Verification items for the finished model (mm, model axes). A direction names the side the tool comes from. Coordinates: 2 decimals unless noted, no trailing zeros. Order: outer loops, then holes, each group sorted by start corner. A loop starts at its lowest first (then second) coordinate and runs counter-clockwise, first axis right, second up.
Q1. Set-up check for faces 4 (the flat face through (0, 8, 49)), 5 (the flat face through (8, 0, 49)), 6 (the flat face through (8, -17, 49)), 7 (the flat face through (-5.05, -19, 49)): record each of +Z, -Z, +X, -X, +Y, -Y from which the full face is reachable in a straight line by a thin tool's end or side.
Q2. Cross-section at A-A, the plane x = 0. Record the boundary of the cut face in (y, z).
Q3. Thickness scan on line 1 (X direction, y = 0, z = 33); line 2 (X direction, y = 18.5, z = 95); line 3 (X direction, y = -8.5, z = 15). Record the ranges inside material, lowest first.
Q4. Depth check by flat-ended pin: P1, Ø8, axis at x = 0.5, z = 16.5, coming from the -Y side; P2, Ø5, axis at x = -15.5, y = 3, coming from the +Z side; P3, Ø5, axis at x = -0.5, z = 18, coming from the -Y side. Enter the tip coordinate at first touch or a pass-through.
Q5. Draft check along X on faces 1 (the flat face through (-19, 5.05, 49)), 2 (the flat face through (-20, 13, 49)), 3 (the flat face through (8.305, -11.134, 50.7)). Enter one of: pulls with the +X half, pulls with the -X half, needs draft (parallel to the pull), parting line crosses it, or undercut.
Autodesk Inventor part; units mm, degrees
ref_plane "YZ Plane" through (0, 0, 0) normal (1, 0, 0) x (0, 1, 0)
ref_plane "XZ Plane" through (0, 0, 0) normal (0, 1, 0) x (-1, 0, 0)
ref_plane "XY Plane" through (0, 0, 0) normal (0, 0, 1) x (1, 0, 0)
sketch "Sketch1" plane through (0, 0, 0) normal (0, 0, 1) x (1, 0, 0)
  arc A0 (0, 5) -> (-5, 0) centre (0, 0) ccw
  line L0 (-5.05, 20.0001) -> (-20, 20.0001)
  line L1 (-20, 20.0001) -> (-20, 5.0501)
  line L2 (-20, 5.0501) -> (-17, 5.0501)
  line L3 (-5.05, 20.0001) -> (-5.05, 17.0001)
  line L4 (0, 8) -> (-3.7572, 8)
  line L5 (-8, 3.7574) -> (-8, 0)
  arc A1 (-15.2929, 11.7574) -> (-17, 11.0503) centre (-16, 11.0503) ccw
  arc A2 (-11.0502, 17.0001) -> (-11.7573, 15.2929) centre (-11.0502, 16.0001) ccw
  line L6 (-17, 5.0501) -> (-17, 11.0503)
  line L7 (-5.05, 17.0001) -> (-11.0502, 17.0001)
  line L8 (-11.7573, 15.2929) -> (-5.4644, 9)
  line L9 (-15.2929, 11.7574) -> (-9, 5.4645)
  line L10 (0, 0) -> (-41.3511, 0) construction
  arc A3 (-5, 0) -> (0, -5) centre (0, 0) ccw
  line L11 (-5.05, -20.0001) -> (-20, -20.0001)
  line L12 (-20, -20.0001) -> (-20, -5.0501)
  line L13 (-20, -5.0501) -> (-17, -5.0501)
  line L14 (-5.05, -20.0001) -> (-5.05, -17.0001)
  line L15 (0, -8) -> (-3.7572, -8)
  line L16 (-8, -3.7574) -> (-8, 0)
  arc A4 (-17, -11.0503) -> (-15.2929, -11.7574) centre (-16, -11.0503) ccw
  arc A5 (-11.7573, -15.2929) -> (-11.0502, -17.0001) centre (-11.0502, -16.0001) ccw
  line L17 (-17, -5.0501) -> (-17, -11.0503)
  line L18 (-5.05, -17.0001) -> (-11.0502, -17.0001)
  line L19 (-11.7573, -15.2929) -> (-5.4644, -9)
  line L20 (-15.2929, -11.7574) -> (-9, -5.4645)
  line L21 (0, 26.9899) -> (0, -26.9183) construction
  arc A6 (0, -5) -> (5, 0) centre (0, 0) ccw
  line L22 (8, -3.7574) -> (8, 0)
  line L23 (15.2929, -11.7574) -> (9, -5.4645)
  line L24 (11.7573, -15.2929) -> (5.4644, -9)
  line L25 (0, -8) -> (3.7572, -8)
  line L26 (5.05, -17.0001) -> (11.0502, -17.0001)
  arc A7 (11.0502, -17.0001) -> (11.7573, -15.2929) centre (11.0502, -16.0001) ccw
  line L27 (5.05, -20.0001) -> (5.05, -17.0001)
  line L28 (5.05, -20.0001) -> (20, -20.0001)
  line L29 (20, -20.0001) -> (20, -5.0501)
  line L30 (20, -5.0501) -> (17, -5.0501)
  line L31 (17, -5.0501) -> (17, -11.0503)
  arc A8 (15.2929, -11.7574) -> (17, -11.0503) centre (16, -11.0503) ccw
  arc A9 (5, 0) -> (0, 5) centre (0, 0) ccw
  line L32 (20, 5.0501) -> (20, 20.0001)
  line L33 (5.05, 20.0001) -> (20, 20.0001)
  line L34 (5.05, 20.0001) -> (5.05, 17.0001)
  line L35 (20, 5.0501) -> (17, 5.0501)
  line L36 (5.4644, 9) -> (11.7573, 15.2929)
  line L37 (9, 5.4645) -> (15.2929, 11.7574)
  line L38 (5.05, 17.0001) -> (11.0502, 17.0001)
  line L39 (17, 5.0501) -> (17, 11.0503)
  arc A10 (11.7573, 15.2929) -> (11.0502, 17.0001) centre (11.0502, 16.0001) ccw
  arc A11 (17, 11.0503) -> (15.2929, 11.7574) centre (16, 11.0503) ccw
  line L40 (-3.7572, 8) -> (-4.7572, 9)
  line L41 (-8, 3.7574) -> (-9, 4.7574)
  line L42 (-9, 4.7574) -> (-9, 5.4645)
  line L43 (-4.7572, 9) -> (-5.4644, 9)
  line L44 (-3.7572, -8) -> (-4.7572, -9)
  line L45 (-8, -3.7574) -> (-9, -4.7574)
  line L46 (-9, -4.7574) -> (-9, -5.4645)
  line L47 (-4.7572, -9) -> (-5.4644, -9)
  line L48 (3.7572, 8) -> (4.7572, 9)
  line L49 (8, 3.7574) -> (9, 4.7574)
  line L50 (9, 4.7574) -> (9, 5.4645)
  line L51 (4.7572, 9) -> (5.4644, 9)
  line L52 (8, -3.7574) -> (9, -4.7574)
  line L53 (9, -4.7574) -> (9, -5.4645)
  line L54 (4.7572, -9) -> (5.4644, -9)
  line L55 (3.7572, -8) -> (4.7572, -9)
  line L56 (0, 8) -> (3.7572, 8)
  line L57 (8, 3.7574) -> (8, 0)
  point P0 (-4.4644, 8)
  point P1 (-8, 4.4645)
  dimension "d0" = 10
  dimension "d3" = 14.95
  dimension "d4" = 14.95
  dimension "d5" = 3
  dimension "d7" = 2
  dimension "d8" = 4
  dimension "d9" = 4
  dimension "d10" = 8.9498
  dimension "d11" = 8.9498
  dimension "d12" = 45
  dimension "d16" = 8
  dimension "d18" = 2.5
  dimension "d19" = 20
  dimension "d21" = 1
  dimension "d24" = 0.5
  dimension "d25" = 0.5
  dimension "d26" = 1
  dimension "d34" = 8
extrude "MK, 40X40" add sketch "Sketch1" along normal blind 100
sketch "Sketch2" plane through (0, 0, 100) normal (0, 0, 1) x (1, 0, 0)
  circle A0 centre (0, 0) radius 5
  line L0 (-9, 5.4645) -> (-15.2929, 11.7574)
  line L1 (-11.7573, 15.2929) -> (-5.4644, 9)
  line L2 (-13.3283, 10.5) -> (-9, 6.1717)
  line L3 (-6.1715, 9) -> (-10.5, 13.3285)
  line L4 (-5.4644, 9) -> (-6.1715, 9)
  line L5 (-5.4644, 9) -> (-4.7572, 9)
  line L6 (-9, 5.4645) -> (-9, 6.1717)
  line L7 (-10.5, 14.0356) -> (-10.5, 13.3285)
  line L8 (-13.3283, 10.5) -> (-14.0355, 10.5)
  line L9 (0, 0) -> (-37.9325, 0) construction
  line L10 (0, 26.9937) -> (0, -28.1119) construction
  line L11 (-13.3283, -10.5) -> (-9, -6.1717)
  line L12 (-6.1715, -9) -> (-10.5, -13.3285)
  line L13 (-5.4644, -9) -> (-6.1715, -9)
  line L14 (-9, -5.4645) -> (-9, -6.1717)
  line L15 (-10.5, -14.0356) -> (-10.5, -13.3285)
  line L16 (-13.3283, -10.5) -> (-14.0355, -10.5)
  line L17 (13.3283, 10.5) -> (9, 6.1717)
  line L18 (6.1715, 9) -> (10.5, 13.3285)
  line L19 (5.4644, 9) -> (6.1715, 9)
  line L20 (9, 5.4645) -> (9, 6.1717)
  line L21 (10.5, 14.0356) -> (10.5, 13.3285)
  line L22 (13.3283, 10.5) -> (14.0355, 10.5)
  line L23 (13.3283, -10.5) -> (14.0355, -10.5)
  line L24 (13.3283, -10.5) -> (9, -6.1717)
  line L25 (9, -5.4645) -> (9, -6.1717)
  line L26 (5.4644, -9) -> (6.1715, -9)
  line L27 (6.1715, -9) -> (10.5, -13.3285)
  line L28 (10.5, -14.0356) -> (10.5, -13.3285)
  line L29 (-14.0355, -10.5) -> (-9, -5.4645)
  line L30 (-15.2929, -11.7574) -> (-9, -5.4645)
  line L31 (-5.4644, -9) -> (-10.5, -14.0356)
  line L32 (-5.4644, -9) -> (-11.7573, -15.2929)
  line L33 (10.5, -14.0356) -> (5.4644, -9)
  line L34 (14.0355, -10.5) -> (9, -5.4645)
  line L35 (9, 5.4645) -> (14.0355, 10.5)
  line L36 (10.5, 14.0356) -> (5.4644, 9)
  dimension "d28" = 4
  dimension "d29" = 0.5
  dimension "d30" = 10.5
  dimension "d31" = 10.5
extrude "Extrusion2" cut sketch "Sketch2" against normal through all contours L0 L8 L2 L6 | L1 L4 L3 L7 | L16 L29 L14 L11 | L13 L31 L15 L12 | L22 L35 L20 L17 | L19 L36 L21 L18 | L24 L25 L34 L23 | L26 L27 L28 L33
equation "\"d4\" = d3"
properties part number "BAR, EXTRUDED ALUM, 40MMX40MM, MK, STD DUTY, 54_01 SERIES" material "Aluminum, 6061-T6"
Check values:
1. face 4: +Z, -Z, +Y
1. face 5: +Z, -Z, +X
1. face 6: +Z, -Z
1. face 7: +Z, -Z, -Y
2. outline: (-8, 0) - (-5, 0) - (-5, 100) - (-8, 100) - close; (5, 0) - (8, 0) - (8, 100) - (5, 100) - close
3. line 1: x = -8 to -5, 5 to 8
3. line 2: x = -20 to -5.05, 5.05 to 20
3. line 3: x = -20 to -17, -11.33 to -4.26, 4.26 to 11.33, 17 to 20
4. P1: stops at y = -8.74
4. P2: passes through
4. P3: stops at y = -8
5. face 1: needs draft
5. face 2: pulls with the -X half
5. face 3: undercut
